Check sheet for the modelled part. Datum: model origin and axes. Units: mm. Face numbers are marked on the shaded views. A direction names the side the tool comes from. Round coordinates to 2 decimals unless told otherwise and drop trailing zeros. Write each loop counter-clockwise with the first axis right and the second up, starting at its lowest first coordinate (ties: lowest second). Pieces come first, ordered by that corner, then holes. Notation, with made-up numbers: M 65.5,-1 L 121.5,-1 A7 cw 121.5,4 Z; hole C 86,18 d6. An arc over 180 degrees is marked long. Put each result on its own line as item: value.
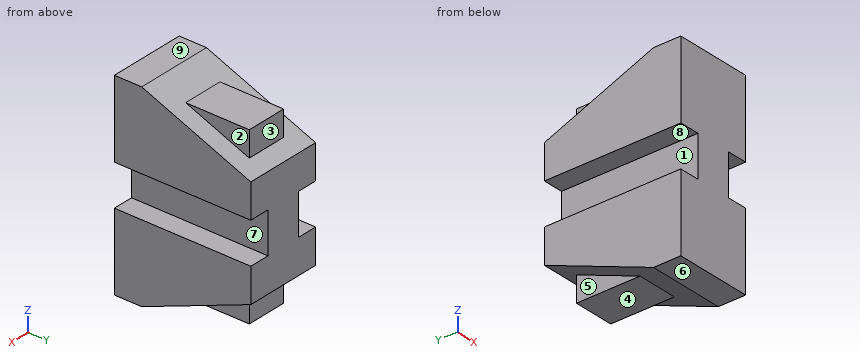
```python
from build123d import *

# Parameters (mm, degrees)
SALIENTE_EXTRUIR2_DEPTH = 17
CROQUIS3_W              = 9
CROQUIS3_H              = 18
CORTAR_EXTRUIR2_DEPTH   = 76.749587458
SALIENTE_EXTRUIR4_DEPTH = 9


with BuildPart() as part:
    # Croquis1 → Saliente-Extruir2 (new, symmetric)
    with BuildSketch(Plane(origin=(0, 0, 0), x_dir=(0, 0, -1), z_dir=(1, 0, 0))):
        Polygon((43, -12), (-43, -12), (-43, 0), (-24, 48), (24, 48), (43, 0), align=None)
    extrude(amount=SALIENTE_EXTRUIR2_DEPTH, both=True)

    # Croquis3 → Cortar-Extruir2 (cut, through all)
    with BuildSketch(Plane(origin=(0, 48, 0), x_dir=(1, 0, 0), z_dir=(0, 1, 0))):
        with Locations((-12.5, 0)):
            Rectangle(CROQUIS3_W, CROQUIS3_H)
        with Locations((12.5, 0)):
            Rectangle(CROQUIS3_W, CROQUIS3_H)
    extrude(amount=-CORTAR_EXTRUIR2_DEPTH, mode=Mode.SUBTRACT)

    # Croquis4 → Saliente-Extruir4 (add, symmetric)
    with BuildSketch(Plane(origin=(0, 0, 0), x_dir=(0, 0, -1), z_dir=(1, 0, 0))):
        Polygon((-38, 12.631578947), (-38, 40.631578947), (-26.916666667, 40.631578947), align=None)
        Polygon((38, 12.631578947), (38, 40.631578947), (26.916666667, 40.631578947), align=None)
    extrude(amount=SALIENTE_EXTRUIR4_DEPTH, both=True)


solid = part.part
```
1. Release check for a two-part mould opening along Z. For the marked faces 6, 7, 8 and 9 record: +Z half, -Z half, draft (parallel to the pull), parting line (faces both ways), or undercut.
Computed values:
face 6: -Z half
face 7: undercut
face 8: undercut
face 9: +Z half
2. Depth check by flat-ended pin: pin 1 Ø9 at (x, z) = (-0.5, 34.5) entering from +Y; pin 2 Ø9 at (y, z) = (33.5, 35) entering from -X; pin 3 Ø7 at (x, y) = (11, 26.5) entering from -Z. Enter the tip coordinate at first touch or a pass-through.
Computed values:
pin 1: stops at y = 40.63
pin 2: stops at x = -9
pin 3: stops at z = -38
3. Cross-section at B-B (y = -5). Enter the section's corners in (x, z).
Computed values:
outline: M -17,-43 L 17,-43 L 17,-9 L 8,-9 L 8,9 L 17,9 L 17,43 L -17,43 L -17,9 L -8,9 L -8,-9 L -17,-9 Z
4. Cross-section at C-C (z = -31.5). Enter the section's corners in (x, y).
Computed values:
outline: M -17,-12 L 17,-12 L 17,29.05 L 9,29.05 L 9,40.63 L -9,40.63 L -9,29.05 L -17,29.05 Z
5. Scan lines: probe 1 along Z at (x, y) = (9.5, -5.5); probe 2 along Y at (x, z) = (6, -30.5); probe 3 along X at (y, z) = (45, -7.5). Record each from-to range of solid material in increasing order.
Computed values:
probe 1: z = -43 to -9, 9 to 43
probe 2: y = -12 to 40.63
probe 3: x = -8 to 8
6. Cross-section at D-D (x = -6). Enter the section's corners in (y, z), then the cut area to 3 significant figures.
Computed values:
outline: M -12,-43 L 0,-43 L 12.63,-38 L 40.63,-38 L 40.63,-26.92 L 48,-24 L 48,24 L 40.63,26.92 L 40.63,38 L 12.63,38 L 0,43 L -12,43 Z
area: 4,560 mm2
7. Access from +Z, -Z, +X, -X, +Y, -Y to the whole of each face (thin tool, end or side, straight path). Record for the marked faces 1, 2, 3, 4 and 5.
Computed values:
face 1: -X, +Y, -Y
face 2: +Z, +X, +Y
face 3: +Z, +X, -X, +Y
face 4: -Z, +X, -X, +Y
face 5: -Z, -X, +Y
8. Cross-section at A-A (x = -15). Enter the section's corners in (y, z), then the cut area to 3 significant figures.
Computed values:
outline: M -12,-43 L 0,-43 L 48,-24 L 48,-9 L -12,-9 Z; M -12,9 L 48,9 L 48,24 L 0,43 L -12,43 Z
area: 3,170 mm2
